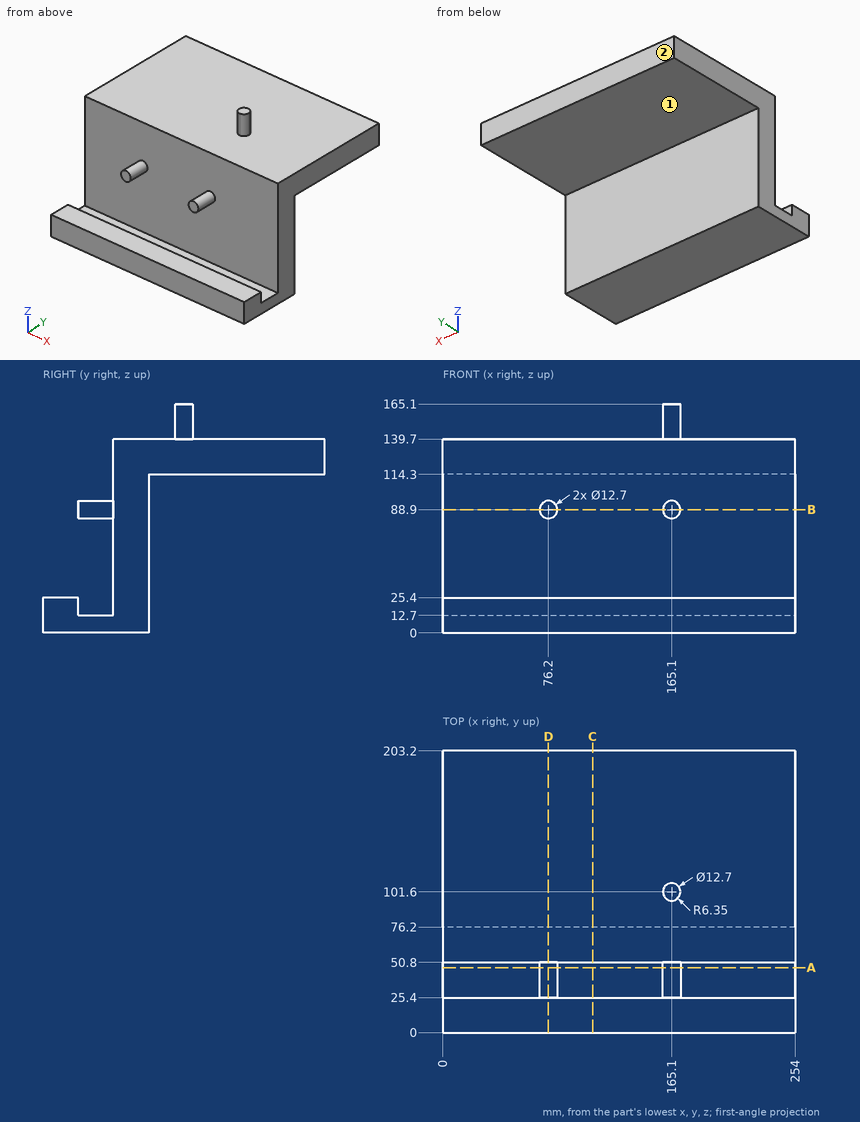
Can you work these out from the drawing? Everything is in mm from the part's minimum corner. A direction names the side the tool comes from. Give positions to 0.01 mm unless a question says otherwise; leave off trailing zeros. Order: outer loops, then holes, each group sorted by start corner. A loop starts at its lowest first (then second) coordinate and runs counter-clockwise, first axis right, second up. Notation, with made-up numbers: M 49.5,46.5 L 56.5,46.5 A9 cw 56.5,56.5 Z; hole C 62.25,48 d3. An arc over 180 degrees is marked long. Use a Markdown table: item, result. Add a question column.
Item 1: If I drill on L1, parallel to Z at x = 184.5, y = 68; L2, parallel to Y at x = 138, z = 64; L3, parallel to Z at x = 105, y = 125, over which ranges is the centre line in solid material (lowest first)? Write a range as [from, to].
Item 2: Suppose I cut it at D-D (x = 76.2). List the corners of the cut face in (y, z) for me.
Item 3: For the marked faces 1 and 2, which set-ups out of +Z, -Z, +X, -X, +Y, -Y let a thin tool reach every point of the face, with its end or its side?
Item 4: Suppose I cut it at B-B (z = 88.9). List the corners of the cut face in (x, y) for me.
Item 5: Will these pins go through, and if not, where does the flat tip stop? pin 1 (20.5 mm diameter, centred on x = 175.5, y = 18.5, fed in from +Z); pin 2 (10 mm diameter, centred on x = 42, z = 74.5, fed in from -Y); pin 3 (10 mm diameter, centred on x = 163.5, z = 92, fed in from -Y).
Item 6: Suppose I cut it at C-C (x = 108). List the corners of the cut face in (y, z) for me.
Item 7: Suppose I cut it at A-A (y = 47). List the corners of the cut face in (x, z) for me, then the cut area to 3 significant figures.
Answer sheet:
| question | item | result |
|---|---|---|
| 1 | L1 | z = [0, 139.7] |
| 1 | L2 | y = [50.8, 76.2] |
| 1 | L3 | z = [114.3, 139.7] |
| 2 | outline | M 0,0 L 76.2,0 L 76.2,114.3 L 203.2,114.3 L 203.2,139.7 L 50.8,139.7 L 50.8,95.25 L 25.4,95.25 L 25.4,82.55 L 50.8,82.55 L 50.8,12.7 L 25.4,12.7 L 25.4,25.4 L 0,25.4 Z |
| 3 | face 1 | -Z, +X, -X, +Y |
| 3 | face 2 | +Z, -Z, +X, -X, +Y |
| 4 | outline | M 0,50.8 L 69.85,50.8 L 69.85,25.4 L 82.55,25.4 L 82.55,50.8 L 158.75,50.8 L 158.75,25.4 L 171.45,25.4 L 171.45,50.8 L 254,50.8 L 254,76.2 L 0,76.2 Z |
| 5 | pin 1 | stops at z = 94.59 |
| 5 | pin 2 | stops at y = 50.8 |
| 5 | pin 3 | stops at y = 25.4 |
| 6 | outline | M 0,0 L 76.2,0 L 76.2,114.3 L 203.2,114.3 L 203.2,139.7 L 50.8,139.7 L 50.8,12.7 L 25.4,12.7 L 25.4,25.4 L 0,25.4 Z |
| 7 | outline | M 0,0 L 254,0 L 254,12.7 L 0,12.7 Z; C 76.2,88.9 d12.7; C 165.1,88.9 d12.7 |
| 7 | area | 3,480 mm² |
